from build123d import *

# Parameters (mm, degrees)
CROQUIS1_W                    = 36.9
CROQUIS1_H                    = 22.4
CROQUIS1_R                    = 2.7
CROQUIS1_R_2                  = 1.99
CROQUIS1_R_3                  = 1.54
SALIENTE_EXTRUIR1_DEPTH       = 9.375
SALIENTE_EXTRUIR2_START       = 9.375
CROQUIS1_3_R                  = 2.7
SALIENTE_EXTRUIR2_DEPTH       = 8.65
SALIENTE_EXTRUIR3_START       = 9.375
CROQUIS1_5_R                  = 1.99
SALIENTE_EXTRUIR3_DEPTH       = 1.77
CROQUIS2_W                    = 8.65
CROQUIS2_H                    = 0.85
CORTAR_EXTRUIR1_DEPTH         = 3.385
CROQUIS1_6_W                  = 4.8
CROQUIS1_6_H                  = 5
CROQUIS1_6_R                  = 1.495
SALIENTE_EXTRUIR4_DEPTH       = 1.4
CROQUIS1_8_W                  = 7.4
CROQUIS1_8_H                  = 9.6
CROQUIS1_8_W_2                = 3.2
CROQUIS1_8_H_2                = 2.55
CROQUIS3_W                    = 22.3
CROQUIS3_H                    = 2.6
CORTAR_EXTRUIR2_DEPTH         = 13.6
CORTAR_EXTRUIR2_DEPTH_BACK    = 13.6
CROQUIS1_10_W                 = 3.2
CROQUIS1_10_H                 = 5.1
SALIENTE_EXTRUIR5_DEPTH       = 11.1
CROQUIS1_11_W                 = 6
CROQUIS1_11_H                 = 19.2
CROQUIS1_11_W_2               = 7.4
CROQUIS1_11_H_2               = 9.6
SALIENTE_EXTRUIR6_DEPTH       = 8
SALIENTE_EXTRUIR6_DEPTH_BACK  = 16.6
TALADRO_ROSCADO_M3X0_51_D     = 2.5
TALADRO_ROSCADO_M3X0_51_DEPTH = 6
TALADRO_ROSCADO_M3X0_51_TIP   = 0.751075774
REDONDEO1_R                   = 3
SALIENTE_EXTRUIR7_START       = 9.375
CROQUIS6_R                    = 3.5
SALIENTE_EXTRUIR7_DEPTH       = 0.55
CHAFL_N1_SIZE                 = 1


with BuildPart() as part:
    # Croquis1 → Saliente-Extruir1 (new body, symmetric)
    with BuildSketch(Plane.XY):
        with Locations((-7.04, 0)):
            Rectangle(CROQUIS1_W, CROQUIS1_H)
        Circle(CROQUIS1_R, mode=Mode.SUBTRACT)
        with Locations((-11, 0)):
            Circle(CROQUIS1_R_2, mode=Mode.SUBTRACT)
        with Locations((-20, 8.7)):
            Circle(CROQUIS1_R_3, mode=Mode.SUBTRACT)
        with Locations((-20, -8.7)):
            Circle(CROQUIS1_R_3, mode=Mode.SUBTRACT)
        Circle(CROQUIS1_R)
        with Locations((-11, 0)):
            Circle(CROQUIS1_R_2)
    extrude(amount=SALIENTE_EXTRUIR1_DEPTH, both=True)

    # Croquis1_3 → Saliente-Extruir2 (add)
    with BuildSketch(Plane.XY.offset(SALIENTE_EXTRUIR2_START)):
        Circle(CROQUIS1_3_R)
    extrude(amount=SALIENTE_EXTRUIR2_DEPTH)

    # Croquis1_5 → Saliente-Extruir3 (add)
    with BuildSketch(Plane.XY.offset(SALIENTE_EXTRUIR3_START)):
        with Locations((-11, 0)):
            Circle(CROQUIS1_5_R)
    extrude(amount=SALIENTE_EXTRUIR3_DEPTH)

    # Croquis2 → Cortar-Extruir1 (cut, symmetric)
    with BuildSketch(Plane(origin=(0, 0, 0), x_dir=(0, 0, -1), z_dir=(1, 0, 0))):
        with Locations((-13.7, 2.275)):
            Rectangle(CROQUIS2_W, CROQUIS2_H)
        with Locations((-13.7, -2.275)):
            Rectangle(CROQUIS2_W, CROQUIS2_H)
    extrude(amount=CORTAR_EXTRUIR1_DEPTH, both=True, mode=Mode.SUBTRACT)

    # Croquis1_6 → Saliente-Extruir4 (add, symmetric)
    with BuildSketch(Plane.XY):
        with Locations((13.81, 0)):
            Rectangle(CROQUIS1_6_W, CROQUIS1_6_H)
        with Locations((13.81, 0)):
            Circle(CROQUIS1_6_R, mode=Mode.SUBTRACT)
    extrude(amount=SALIENTE_EXTRUIR4_DEPTH, both=True)

    # Croquis1_8 → Revoluci_n1 (revolve)
    with BuildSketch(Plane.XY):
        Polygon((-30.19, 0), (-25.49, 0), (-25.49, 11.2), (-35.44, 11.2), (-35.44, 12.6), (-57.74, 12.6), (-57.74, 9.6), (-50.34, 9.6), (-50.34, 0), (-33.39, 0), (-33.39, 2.55), (-30.19, 2.55), align=None)
        with Locations((-54.04, 4.8)):
            Rectangle(CROQUIS1_8_W, CROQUIS1_8_H)
        with Locations((-31.79, 1.275)):
            Rectangle(CROQUIS1_8_W_2, CROQUIS1_8_H_2)
    revolve(axis=Axis((-25.49, 0, 0), (-1, 0, 0)))

    # Croquis3 → Cortar-Extruir2 (cut, two sides)
    with BuildSketch(Plane(origin=(0, 0, 0), x_dir=(1, 0, 0), z_dir=(0, 1, 0))) as cortar_extruir2_sk:
        Polygon((-35.44, 10), (-35.44, 9.375), (-25.49, 9.375), (-25.49, 11.2), (-35.44, 11.2), align=None)
        with Locations((-46.59, 11.3)):
            Rectangle(CROQUIS3_W, CROQUIS3_H)
        with Locations((-46.59, -11.3)):
            Rectangle(CROQUIS3_W, CROQUIS3_H)
        Polygon((-25.49, -9.375), (-35.44, -9.375), (-35.44, -10), (-35.44, -11.2), (-25.49, -11.2), align=None)
    extrude(amount=CORTAR_EXTRUIR2_DEPTH, mode=Mode.SUBTRACT)
    extrude(cortar_extruir2_sk.sketch, amount=-CORTAR_EXTRUIR2_DEPTH_BACK, mode=Mode.SUBTRACT)

    # Croquis1_10 → Saliente-Extruir5 (add, symmetric)
    with BuildSketch(Plane.XY):
        with Locations((-31.79, 0)):
            Rectangle(CROQUIS1_10_W, CROQUIS1_10_H)
    extrude(amount=SALIENTE_EXTRUIR5_DEPTH, both=True)

    # Croquis1_11 → Saliente-Extruir6 (add, two sides)
    with BuildSketch(Plane.XY) as saliente_extruir6_sk:
        with Locations((-60.74, 0)):
            Rectangle(CROQUIS1_11_W, CROQUIS1_11_H)
        with Locations((-54.04, 4.8)):
            Rectangle(CROQUIS1_11_W_2, CROQUIS1_11_H_2)
        with Locations((-54.04, -4.8)):
            Rectangle(CROQUIS1_11_W_2, CROQUIS1_11_H_2)
    extrude(amount=SALIENTE_EXTRUIR6_DEPTH)
    extrude(saliente_extruir6_sk.sketch, amount=-SALIENTE_EXTRUIR6_DEPTH_BACK)

    # Taladro roscado M3x0.51
    with Locations(Plane.XY.offset(18.025)):
        with Locations((0, 0)):
            Hole(TALADRO_ROSCADO_M3X0_51_D / 2, depth=TALADRO_ROSCADO_M3X0_51_DEPTH)
            with Locations((0, 0, -(TALADRO_ROSCADO_M3X0_51_DEPTH + TALADRO_ROSCADO_M3X0_51_TIP / 2))):  # 118° drill point
                Cone(0, TALADRO_ROSCADO_M3X0_51_D / 2, TALADRO_ROSCADO_M3X0_51_TIP, mode=Mode.SUBTRACT)

    # Redondeo1
    redondeo1_edges = [part.edges().sort_by_distance(p)[0] for p in [
        (11.41, 11.2, 0),
        (11.41, -11.2, 0),
    ]]
    fillet(redondeo1_edges, radius=REDONDEO1_R)

    # Croquis6 → Saliente-Extruir7 (add)
    with BuildSketch(Plane.XY.offset(SALIENTE_EXTRUIR7_START)):
        Circle(CROQUIS6_R)
    extrude(amount=SALIENTE_EXTRUIR7_DEPTH)

    # Chafl_n1
    chafl_n1_edges = [part.edges().sort_by_distance(p)[0] for p in [
        (-33.39, 0, 11.1),
    ]]
    chamfer(chafl_n1_edges, length=CHAFL_N1_SIZE)


solid = part.part
Geometry: final body of the model. Coordinates: model frame, mm. A direction names the side the tool comes from. Give positions to 0.01 mm unless a question says otherwise; leave off trailing zeros. Loops run counter-clockwise (first coordinate to the right, second up) from the corner with the lowest first, then second, coordinate; pieces in that order, holes last. Notation, with made-up numbers: (80.5, 0) - (137.5, 0) arc R22 cw to (137.5, 33) - close; hole circle Ø2 at (2.25, 61). An arc over 180 degrees is marked (long way). One line per question, with ' | ' between items. Start each with the question number.
(1) Pull-direction query (X, two-part tool) for faces 5 (the flat face through (-59, -9.6, -7)), 6 (the flat face through (16.21, 0, 0)), 7 (the flat face through (-32, 2.55, 10)), 8 (the flat face through (-25.49, 10, -7)); classes: released by +X, released by -X, zero draft, split by the parting line, or undercut.
(2) Contact query for flat-ended pins moving along their axis: pin 1 (3 mm diameter, centred on x = -0.5, z = 14.5, fed in from -Y); pin 2 (4 mm diameter, centred on x = -20, y = 8.7, fed in from +Z) (3 decimals); pin 3 (1.1 mm diameter, centred on x = -31.5, y = 0, fed in from +Z); pin 4 (6.5 mm diameter, centred on x = -55.5, z = -1, fed in from +Y). Output: stop coordinate, or through.
(3) Ray query, line 1 (Y direction, x = -20, z = 0); line 2 (X direction, y = 0, z = 14.2); line 3 (Y direction, x = 13.81, z = 0.4) (3 decimals). Return the intervals inside material, ascending. Write a range as from..to.
(4) Section query D-D on x = -11. Return loops of the section in (y, z) (3 decimals).
(5) Reachability of faces 1 (the cylindrical face through (0.27, -1.22, 14.98)), 2 (the flat face through (12, 0, 1.4)), 3 (the flat face through (-32, 0, -11.1)), 4 (the flat face through (14, 2.5, 0)) from +Z, -Z, +X, -X, +Y, -Y: full face, straight path, thin tool, end or side. Return the list, or none.
(6) Section query B-B on y = -5. Return loops of the section in (x, z) (3 decimals).
(7) Section query A-A on x = -20. Return loops of the section in (y, z) (3 decimals).
(8) Section query C-C on z = 14.5. Return loops of the section in (x, y), then the cut area to 3 significant figures.
The answers:
1) face 5: zero draft | face 6: released by +X | face 7: undercut | face 8: undercut
2) pin 1: y = -1.85 | pin 2: z = 9.375 | pin 3: z = 11.1 | pin 4: y = 12.6
3) line 1: -11.2..-10.24, -7.16..7.16, 10.24..11.2 | line 2: -2.7..-1.25, 1.25..2.7 | line 3: -2.5..-1.495, 1.495..2.5
4) outline: (-11.2, -9.375) - (11.2, -9.375) - (11.2, 9.375) - (1.99, 9.375) - (1.99, 11.145) - (-1.99, 11.145) - (-1.99, 9.375) - (-11.2, 9.375) - close
5) face 1: +Z | face 2: +Z, +X, +Y, -Y | face 3: -Z, +X, +Y, -Y | face 4: +Z, -Z, +X, +Y
6) outline: (-63.74, -16.6) - (-50.34, -16.6) - (-50.34, -10) - (-35.44, -10) - (-35.44, -9.375) - (11.41, -9.375) - (11.41, 9.375) - (-35.44, 9.375) - (-35.44, 10) - (-57.74, 10) - (-57.74, 8) - (-63.74, 8) - close
7) outline: (-11.2, -9.375) - (-10.24, -9.375) - (-10.24, 9.375) - (-11.2, 9.375) - close; (-7.16, -9.375) - (7.16, -9.375) - (7.16, 9.375) - (-7.16, 9.375) - close; (10.24, -9.375) - (11.2, -9.375) - (11.2, 9.375) - (10.24, 9.375) - close
8) outline: (-1.97, -1.85) - (1.97, -1.85) arc R2.7 ccw to (1.97, 1.85) - (-1.97, 1.85) arc R2.7 ccw to start; hole circle Ø2.5 at (0, 0) | area: 13.4 mm2
